from build123d import *

# Parameters (mm, degrees)
BOX_W     = 40
BOX_H     = 40
BOX_DEPTH = 3
FILLET_R  = 3


with BuildPart() as con001:
    # Cone001 → Cone001 (revolve)
    with BuildSketch(Plane(origin=(0, 0, -4), x_dir=(1, 0, 0), z_dir=(0, -1, 0))):
        Polygon((0, 0), (15, 0), (3, 44), (0, 44), align=None)
    revolve(axis=Axis((0, 0, -4), (0, 0, 1)))


with BuildPart() as con:
    # Cone → Cone (revolve)
    with BuildSketch(Plane.XZ):
        Polygon((0, 0), (16, 0), (4, 40), (0, 40), align=None)
    revolve(axis=Axis((0, 0, 0), (0, 0, 1)))


with BuildPart() as cut:
    # Box → Box (new body)
    with BuildSketch(Plane.XY):
        with Locations((20, 20)):
            Rectangle(BOX_W, BOX_H)
    extrude(amount=BOX_DEPTH)

    # Fillet
    fillet_edges = [cut.edges().sort_by_distance(p)[0] for p in [
        (0, 0, 1.5),
        (0, 40, 1.5),
        (40, 0, 1.5),
        (40, 40, 1.5),
    ]]
    fillet(fillet_edges, radius=FILLET_R)


with BuildPart() as cut_1:
    # Fillet placement: moved
    add(cut.part.moved(Location((-20, -20, -3))))

    # Fusion: union Con
    add(con.part)

    # Cut: cut Con001
    add(con001.part, mode=Mode.SUBTRACT)


solid = cut_1.part
Read the model definition and answer for the solid it produces. Units are mm, in the model's axes. A direction names the side the tool comes from. Give positions to 0.01 mm unless a question says otherwise; leave off trailing zeros. Write each loop counter-clockwise with the first axis right and the second up, starting at its lowest first coordinate (ties: lowest second). Pieces come first, ordered by that corner, then holes. Notation, with made-up numbers: (65.5, 63) - (71.5, 63) arc R33 ccw to (71.5, 91) - close; hole circle Ø10 at (39.5, -18). An arc over 180 degrees is marked (long way). Answer in a Markdown table with one row per item. Add a question column.
Item 1: Section D-D, the plane z = 13.5 is taken. Write down the section's boundary in (x, y).
Item 2: Find the intervals of material crossed by L1, parallel to Z at x = -13.5, y = 12; L2, parallel to X at y = -4, z = 8; L3, parallel to Y at x = -8, z = 1.5, in increasing order.
Item 3: Section C-C, the plane z = 18 is taken. Write down the section's boundary in (x, y).
Item 4: Flat-ended cylindrical pins translate along their axes: P1, Ø6, axis at y = 12, z = 4.5, coming from the -X side; P2, Ø2, axis at y = -7.5, z = 24.5, coming from the +X side; P3, Ø6, axis at y = 6.5, z = 24, coming from the -X side. Find the tip coordinate at first contact, or state that the pin passes through.
Item 5: Determine the mould class of faces 3 (the face through (20, 0, -2)), 4 (the face through (-19.14, -19.1, -1.48)), 5 (the face through (0, 20, -2)), 6 (the face through (8.376, 2.638, 18.801)) for opening direction X: pulls with the +X half, pulls with the -X half, needs draft (parallel to the pull), parting line crosses it, or undercut.
Item 6: Section A-A, the plane x = 0 is taken. Write down the section's boundary in (y, z), and give its area (3 significant figures).
Item 7: A tool of negligible diameter and unlimited length cuts with its end or side. For faces 1 (the face through (0, -20, -2)), 2 (the face through (-9, 14, 0)), from which of +Z, -Z, +X, -X, +Y, -Y can it reach the whole face along a straight path? Write none if from no direction.
Recorded:
| question | item | result |
|---|---|---|
| 1 | outline | circle Ø23.9 at (0, 0); hole circle Ø20.45 at (0, 0) |
| 2 | L1 | z = -3 to 0 |
| 2 | L2 | x = -13 to -11.02, 11.02 to 13 |
| 2 | L3 | y = -13.33 to -10.87, 10.87 to 13.33 |
| 3 | outline | circle Ø21.2 at (0, 0); hole circle Ø18 at (0, 0) |
| 4 | P1 | stops at x = -11.82 |
| 4 | P2 | stops at x = 5.79 |
| 4 | P3 | stops at x = -8.39 |
| 5 | face 3 | pulls with the +X half |
| 5 | face 4 | pulls with the -X half |
| 5 | face 5 | needs draft |
| 5 | face 6 | undercut |
| 6 | outline | (-20, -3) - (-14.73, -3) - (-3, 40) - (-4, 40) - (-16, 0) - (-20, 0) - close; (3, 40) - (14.73, -3) - (20, -3) - (20, 0) - (16, 0) - (4, 40) - close |
| 6 | area | 158 mm2 |
| 7 | face 1 | +Z, -Z, +X, -X, -Y |
| 7 | face 2 | +Z |
